Check sheet for the modelled part. Datum: model origin and axes. Units: mm. A direction names the side the tool comes from. Coordinates: 2 decimals unless noted, no trailing zeros. Write each loop counter-clockwise with the first axis right and the second up, starting at its lowest first coordinate (ties: lowest second). Pieces come first, ordered by that corner, then holes. Notation, with made-up numbers: (-0.5, 64.25) - (25.5, 64.25) arc R16 ccw to (25.5, 79.25) - close; hole circle Ø9 at (6.25, -1.75). An arc over 180 degrees is marked (long way). Use one line per item in the form item = value. Start each with the question number.
1. Cross-section at B-B on x = 0. Record the boundary of the cut face in (y, z), then the cut area to 3 significant figures.
2. Tool access check on faces 4 (the face through (-15, 9, 7)), 5 (the face through (6.131, -7.535, 4.534)), 6 (the face through (12, 1, 6)). Record the directions out of +Z, -Z, +X, -X, +Y, -Y that give a thin tool (end or side, any length) a straight path to the whole face; none if there is none.
3. Cross-section at C-C on x = -5. Record the boundary of the cut face in (y, z), then the cut area to 3 significant figures.
4. Go/stop test with a flat-tipped pin: pin 1 Ø3.5 at (x, z) = (10, 7.5) entering from -Y. Record where the tip stops, or that it passes through.
5. Draft check along X on faces 1 (the face through (16, 5, 7)), 2 (the face through (-6, 0, 7)), 3 (the face through (-15, -9, 7)). Enter one of: +X half, -X half, draft (parallel to the pull), parting line (faces both ways), or undercut.
6. Cross-section at A-A on x = 10. Record the boundary of the cut face in (y, z) (3 decimals).
7. Scan lines: line 1 along Y through (x, z) = (13, 13.5); line 2 along Y through (x, z) = (0, 6.5); line 3 along X through (y, z) = (-3.25, 5). Record each from-to range of solid material in increasing order.
```python
from build123d import *

# Parameters (mm, degrees)
F1_DEPTH = 15
F2_SIZE2 = 2
F2_SIZE  = 2
F3_R     = 2.75
F4_DEPTH = 10
F6_D     = 4.2
F5_R     = 4.875
F5_R_2   = 2.75
F7_DEPTH = 5
F9_D     = 0.5


with BuildPart() as f1:
    # F0 (on Top) → F1 (new body)
    with BuildSketch(Plane.XY):
        with BuildLine():
            ThreePointArc((5.9160797831, -1), (-6, 0), (5.9160797831, 1))
            Line((5.9160797831, 1), (16, 1))
            Line((16, 1), (16, 10))
            Line((16, 10), (-16, 10))
            Line((-16, 10), (-16, -10))
            Line((-16, -10), (16, -10))
            Line((16, -10), (16, -1))
            Line((16, -1), (5.9160797831, -1))
        make_face()
    extrude(amount=F1_DEPTH)

    # F2
    f2_edges = [f1.edges().sort_by_distance(p)[0] for p in [
        (-16, 10, 7.5),
        (-16, -10, 7.5),
    ]]
    chamfer(f2_edges, length=F2_SIZE, length2=F2_SIZE2)

    # F3 (on face) → F4 (cut)
    with BuildSketch(Plane.XZ.offset(10)):
        with Locations((10, 7.5)):
            Circle(F3_R)
    extrude(amount=-F4_DEPTH, mode=Mode.SUBTRACT)

    # F6 (through all)
    with Locations(Plane.XZ.offset(10)):
        with Locations((10, 7.5)):
            Hole(F6_D / 2)

    # F5 (on face) → F7 (cut)
    with BuildSketch(Plane.XZ.offset(10)):
        with Locations((10, 7.5)):
            Circle(F5_R)
        with Locations((10, 7.5)):
            Circle(F5_R_2, mode=Mode.SUBTRACT)
    extrude(amount=-F7_DEPTH, mode=Mode.SUBTRACT)

    # F9 (through all)
    with Locations(Plane(origin=(-16, 0, 0), x_dir=(0, -1, 0), z_dir=(-1, 0, 0))):
        with Locations((0, 7.5)):
            Hole(F9_D / 2)


solid = f1.part
```
Final values:
q1.outline = (-10, 0) - (-6, 0) - (-6, 15) - (-10, 15) - close; (6, 0) - (10, 0) - (10, 15) - (6, 15) - close
q1.area = 120 mm²
q2.face_4 = +Z, -Z, -X, +Y
q2.face_5 = -Y
q2.face_6 = +Z, -Z, +X
q3.outline = (-10, 0) - (-3.32, 0) - (-3.32, 15) - (-10, 15) - close; (3.32, 0) - (10, 0) - (10, 15) - (3.32, 15) - close
q3.area = 201 mm²
q4.pin_1 = through
q5.face_1 = +X half
q5.face_2 = undercut
q5.face_3 = -X half
q6.outline = (-10, 0) - (-1, 0) - (-1, 4.75) - (-5, 4.75) - (-5, 2.625) - (-10, 2.625) - close; (-10, 12.375) - (-5, 12.375) - (-5, 10.25) - (-1, 10.25) - (-1, 15) - (-10, 15) - close; (1, 0) - (10, 0) - (10, 5.4) - (1, 5.4) - close; (1, 9.6) - (10, 9.6) - (10, 15) - (1, 15) - close
q7.line_1 = -10 to -1, 1 to 10
q7.line_2 = -10 to -6, 6 to 10
q7.line_3 = -16 to -5.04, 5.04 to 8.85, 11.15 to 16
